Geometry: final body of the model. Coordinates: model frame, mm. Face numbers are marked on the shaded views. A direction names the side the tool comes from. Give positions to 0.01 mm unless a question says otherwise; leave off trailing zeros. Order: outer loops, then holes, each group sorted by start corner. A loop starts at its lowest first (then second) coordinate and runs counter-clockwise, first axis right, second up. Notation, with made-up numbers: (33.5, -4) - (64.5, -4) arc R24 ccw to (64.5, 32) - close; hole circle Ø9 at (56, 3.5). An arc over 180 degrees is marked (long way). One line per item, written item: value.
```python
from build123d import *

# Parameters (mm, degrees)
F1_DEPTH = 25.4
F2_W     = 12.7
F2_H     = 12.7
F3_DEPTH = 63.5
F4_DEPTH = 76.2
F6_DEPTH = 12.7


with BuildPart() as f1:
    # F0 (on Top) → F1 (new body)
    with BuildSketch(Plane.XY):
        Polygon((-82.4187099934, -81.6961601377), (82.4187099934, -81.6961601377), (82.4187099934, 81.6961601377), align=None)
    extrude(amount=F1_DEPTH)

    # F2 (on face) → F3 (join)
    with BuildSketch(Plane.XY.offset(25.4)):
        Polygon((37.3201792488, 36.9930000181), (28.3004730998, 28.0523679941), (37.2411051238, 19.0326618452), (46.2608112727, 27.9732938691), align=None)
        Polygon((82.4187099934, 56.2961601377), (-57.0187099934, -81.6961601377), (-31.6187099934, -81.6961601377), (-18.9187099934, -81.6961601377), (82.4187099934, 18.1961601377), (82.4187099934, 30.8961601377), (82.4187099934, 43.5961601377), align=None)
        with Locations((76.0687099934, -13.5538398623)):
            Rectangle(F2_W, F2_H)
        with Locations((25.5312900066, -75.3461601377)):
            Rectangle(F2_W, F2_H)
        Polygon((-28.293198853, -28.0451575193), (-37.3201792488, -36.9930000181), (-28.3795472248, -46.012706167), (-19.3526364396, -37.0793483618), align=None)
    extrude(amount=F3_DEPTH)

    # F4 (cut): a face of the model
    f4_faces = [f1.faces().sort_by_distance(p)[0] for p in [
        (21.8407092905, -21.5998593386, 88.9),
    ]]
    extrude(f4_faces, amount=-F4_DEPTH, mode=Mode.SUBTRACT)

    # F5 (on face) → F6 (join)
    with BuildSketch(Plane.XY.offset(25.4)):
        Polygon((82.4187099934, 18.1961601377), (-18.9187099934, -81.6961601377), (-8.7587099934, -81.6961601377), (82.4187099934, 8.1810445552), align=None)
    extrude(amount=-F6_DEPTH)


solid = f1.part
```
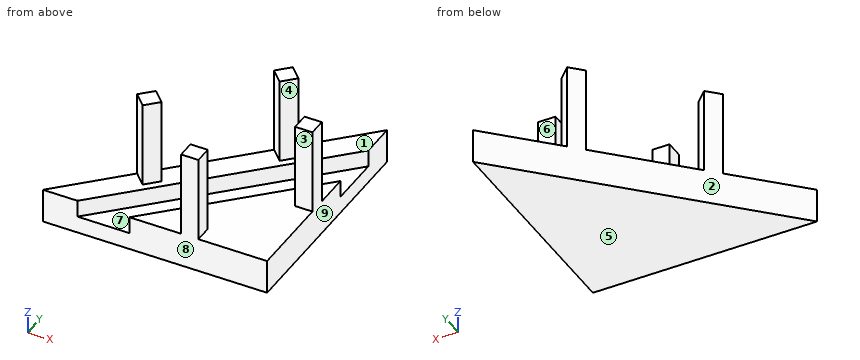
1) Section B-B, the plane x = 55. Return loops of the section in (y, z), then the cut area to 3 significant figures.
Answers below:
outline: (-81.7, 0) - (54.52, 0) - (54.52, 25.4) - (29.16, 25.4) - (29.16, 12.7) - (-8.83, 12.7) - (-8.83, 25.4) - (-81.7, 25.4) - close
area: 2,980 mm^2
2) Section A-A, the plane z = 62. Return loops of the section in (x, y), then the cut area to 3 significant figures.
Answers below:
outline: (-37.32, -36.99) - (-28.38, -46.01) - (-19.35, -37.08) - (-28.29, -28.05) - close; (19.18, -81.7) - (31.88, -81.7) - (31.88, -69) - (19.18, -69) - close; (28.3, 28.05) - (37.24, 19.03) - (46.26, 27.97) - (37.32, 36.99) - close; (69.72, -19.9) - (82.42, -19.9) - (82.42, -7.2) - (69.72, -7.2) - close
area: 645 mm^2
3) Section C-C, the plane y = 5. Return loops of the section in (x, z), then the cut area to 3 significant figures.
Answers below:
outline: (5.04, 0) - (82.42, 0) - (82.42, 25.4) - (69.03, 25.4) - (69.03, 12.7) - (30.59, 12.7) - (30.59, 25.4) - (5.04, 25.4) - close
area: 1,480 mm^2
4) Section D-D, the plane y = -13.5. Return loops of the section in (x, z), then the cut area to 3 significant figures.
Answers below:
outline: (-13.62, 0) - (82.42, 0) - (82.42, 88.9) - (69.72, 88.9) - (69.72, 25.4) - (50.26, 25.4) - (50.26, 12.7) - (11.89, 12.7) - (11.89, 25.4) - (-13.62, 25.4) - close
area: 2,760 mm^2
5) Material intervals for line 1 along Z through (x, y) = (63, -9); line 2 along Y through (x, z) = (30, 57.5); line 3 along X through (y, z) = (-73.5, 37), sorted ascending.
Answers below:
line 1: 0 to 25.4
line 2: -81.7 to -69, 26.34 to 29.74
line 3: 19.18 to 31.88
6) Set-up query: the marked faces 1, 2, 3, 4 and 5. Return all of +Z, -Z, +X, -X, +Y, -Y with unobstructed straight access to the full face (end or side cutting, diameter ignored); none if empty.
Answers below:
face 1: +Z
face 2: +Z, -Z, -X, +Y
face 3: +Z, +X, -X, -Y
face 4: +Z, +X, -Y
face 5: -Z, +X, -X, +Y, -Y
7) First-contact query: pin 1 (4 mm diameter, centred on y = -75.5, z = 58, fed in from +X); pin 2 (10 mm diameter, centred on y = -3.5, z = 68.5, fed in from -X); pin 3 (6.5 mm diameter, centred on x = 79, z = 54, fed in from -Y). Flat tips, straight axial feed; report the tip coordinate or a pass-through.
Answers below:
pin 1: x = 31.88
pin 2: x = 69.72
pin 3: y = -19.9
8) Mould query, pull axis Y, two halves, no side actions, for the marked faces 6, 7, 8 and 9. Classes: released by +Y, released by -Y, zero draft, split by the parting line, or undercut.
Answers below:
face 6: released by +Y
face 7: undercut
face 8: released by -Y
face 9: zero draft
